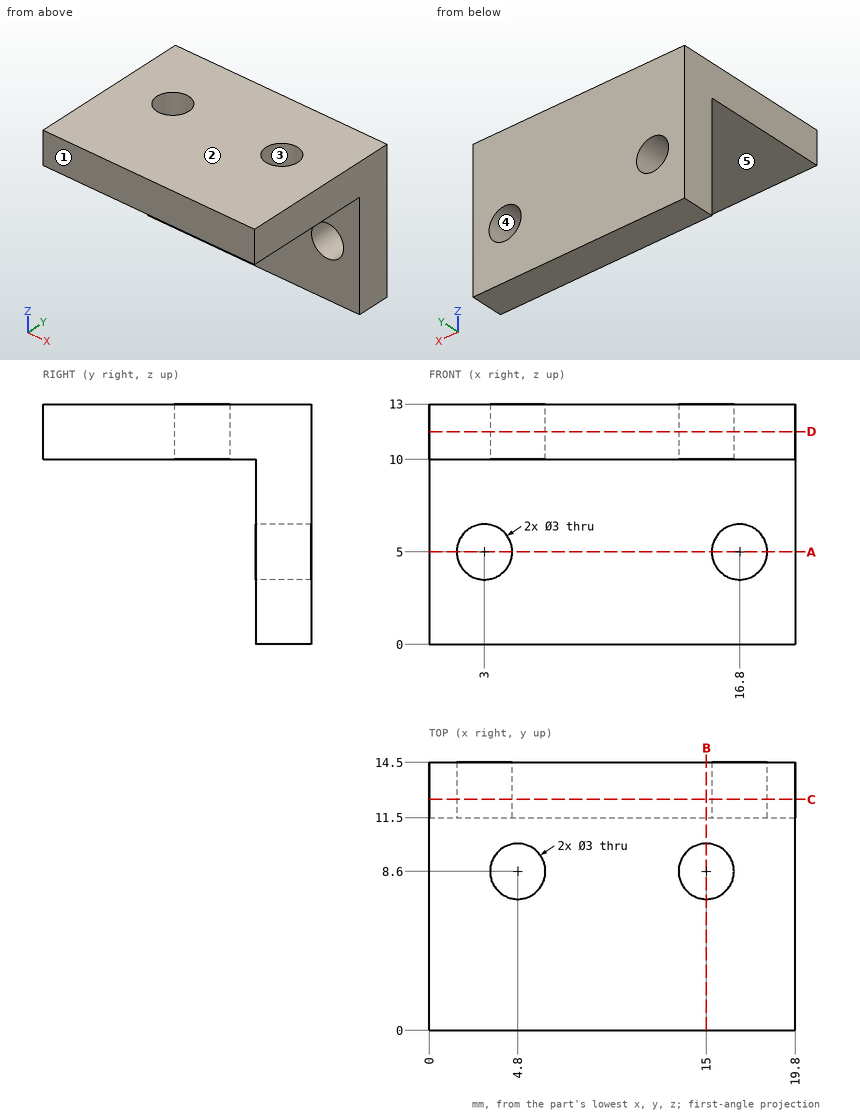
Geometry check sheet. Reference: drawing and pictorial views, mm from the part's lowest x, y, z. A direction names the side the tool comes from. Coordinates: 2 decimals unless noted, no trailing zeros. Write each loop counter-clockwise with the first axis right and the second up, starting at its lowest first coordinate (ties: lowest second). Pieces come first, ordered by that corner, then holes. Notation, with made-up numbers: (53.25, 30.25) - (64.25, 30.25) arc R28 cw to (64.25, 64.25) - close; hole circle Ø3 at (77.5, -18). An arc over 180 degrees is marked (long way). One line per question, with ' | ' between items. Start each with the question number.
1. Section check D-D (z = 11.5). Enter the section's corners in (x, y).
2. Access from +Z, -Z, +X, -X, +Y, -Y to the whole of each face (thin tool, end or side, straight path). Record for the marked faces 4 and 5.
3. Material ranges on line 1 along Y through (x, z) = (15, 12.1); line 2 along Z through (x, y) = (3, 13.8); line 3 along Z through (x, y) = (1.75, 11), recorded low to high.
4. Section check B-B (x = 15). Enter the section's corners in (y, z), plus the area to 3 significant figures.
5. Draft check along Y on the marked faces 1, 2 and 3. Enter one of: released by +Y, released by -Y, zero draft, split by the parting line, or undercut.
6. Gauge pin test, flat ends, axial feed: P1, Ø2.5, axis at x = 4.8, y = 8.6, coming from the -Z side; P2, Ø5, axis at x = 12.5, z = 2.5, coming from the -Y side; P3, Ø1.5, axis at x = 9.5, y = 10, coming from the -Z side; P4, Ø5, axis at x = 16.8, z = 5, coming from the +Y side. Record the tip position at first contact, or that the pin passes through.
7. Section check C-C (y = 12.5). Enter the section's corners in (x, z), plus the area to 3 significant figures.
8. Section check A-A (z = 5). Enter the section's corners in (x, y), plus the area to 3 significant figures.
Computed values:
1) outline: (0, 0) - (19.8, 0) - (19.8, 14.5) - (0, 14.5) - close; hole circle Ø3 at (4.8, 8.6); hole circle Ø3 at (15, 8.6)
2) face 4: +Y, -Y | face 5: -Z, +X, -X, -Y
3) line 1: 0 to 7.1, 10.1 to 14.5 | line 2: 0 to 3.5, 6.5 to 13 | line 3: 10 to 13
4) outline: (0, 10) - (7.1, 10) - (7.1, 13) - (0, 13) - close; (10.1, 10) - (11.5, 10) - (11.5, 0) - (14.5, 0) - (14.5, 13) - (10.1, 13) - close | area: 64.5 mm²
5) face 1: released by -Y | face 2: zero draft | face 3: undercut
6) P1: through | P2: y = 11.5 | P3: z = 10 | P4: y = 14.5
7) outline: (0, 0) - (19.8, 0) - (19.8, 13) - (0, 13) - close; hole circle Ø3 at (3, 5); hole circle Ø3 at (16.8, 5) | area: 243 mm²
8) outline: (0, 11.5) - (1.5, 11.5) - (1.5, 14.5) - (0, 14.5) - close; (4.5, 11.5) - (15.3, 11.5) - (15.3, 14.5) - (4.5, 14.5) - close; (18.3, 11.5) - (19.8, 11.5) - (19.8, 14.5) - (18.3, 14.5) - close | area: 41.4 mm²
